CAD build for the part. Positions are in the model's coordinates, mm. A direction names the side the tool comes from. Coordinates: 2 decimals unless noted, no trailing zeros. Write each loop counter-clockwise with the first axis right and the second up, starting at its lowest first coordinate (ties: lowest second). Pieces come first, ordered by that corner, then holes. Notation, with made-up numbers: (-38.75, 65) - (6.25, 65) arc R24 ccw to (6.25, 76) - close; hole circle Ø4 at (-37.5, 79). An arc over 180 degrees is marked (long way). One line per question, with ' | ' between items. Start each with the question number.
1. Which spindle directions (+Z, -Z, +X, -X, +Y, -Y) get a long thin tool onto all of the face, cutting with end or side? Do faces 1 (the flat face through (-90, 25, -5)), 2 (the flat face through (8, 10, -55)), 3 (the flat face through (40, 5, -26)), 4 (the flat face through (-40, 5, -26)), 5 (the flat face through (90, 25, -5)). Say none if no direction does.
2. Flat gauge pins, fed straight in: P1, Ø12, axis at x = -20.5, z = -42, coming from the +Y side; P2, Ø6, axis at x = -5, z = -49.5, coming from the +Y side; P3, Ø3, axis at y = 4.5, z = -26.5, coming from the +X side; P4, Ø4, axis at x = -24.5, y = 17, coming from the -Z side. Where does each tip first touch, or does it go through?
3. Probe line 1 (X direction, y = 7, z = -42); line 2 (Z direction, x = 51.5, y = 28.5); line 3 (Y direction, x = 2, z = -70). List the from-to ranges inside material, lowest first.
4. Band-saw the part on A-A, the plane x = 0. Write the cut outline in (y, z), then the cut area to 3 significant figures.
5. Band-saw the part on B-B, the plane y = 7. Write the cut outline in (x, z).
6. Band-saw the part on D-D, the plane x = 24. Write the cut outline in (y, z).
7. Band-saw the part on C-C, the plane z = -34. Write the cut outline in (x, y).
8. Two-plate mould, pull along Z, no slides. Class faces 6 (the flat face through (-1, 25, 0)), 7 (the flat face through (-1, 50, -5)), 8 (the cylindrical face through (0.88, 4.93, -82.49)), 9 (the cylindrical face through (8.45, 4.93, -51.71)): +Z half, -Z half, draft (parallel to the pull), parting line (faces both ways), or undercut.
from build123d import *

# Parameters (mm, degrees)
SKETCH1_R           = 12.5
BOSS_EXTRUDE1_DEPTH = 10
SKETCH2_W           = 180
SKETCH2_H           = 50
BOSS_EXTRUDE2_DEPTH = 10


with BuildPart() as part:
    # Sketch1 → Boss-Extrude1 (new body)
    with BuildSketch(Plane(origin=(0, 0, 0), x_dir=(1, 0, 0), z_dir=(0, 1, 0))):
        with BuildLine():
            Line((-40, 0), (40, 0))
            Line((40, 0), (40, 42.5))
            ThreePointArc((40, 42.5), (0, 82.5), (-40, 42.5))
            Line((-40, 42.5), (-40, 0))
        make_face()
        with Locations(Location((0, 42.5, 0), (0, 0, 270))):
            Circle(SKETCH1_R, mode=Mode.SUBTRACT)
    extrude(amount=BOSS_EXTRUDE1_DEPTH)

    # Sketch2 → Boss-Extrude2 (add)
    with BuildSketch(Plane.XY):
        with Locations((0, 25)):
            Rectangle(SKETCH2_W, SKETCH2_H)
    extrude(amount=-BOSS_EXTRUDE2_DEPTH)


solid = part.part
Filled in:
1) face 1: +Z, -Z, -X, +Y, -Y | face 2: -Z, +X, -X, +Y | face 3: -Z, +X, +Y, -Y | face 4: -Z, -X, +Y, -Y | face 5: +Z, -Z, +X, +Y, -Y
2) P1: stops at y = 10 | P2: passes through | P3: stops at x = 40 | P4: stops at z = -10
3) line 1: x = -40 to -12.49, 12.49 to 40 | line 2: z = -10 to 0 | line 3: y = 0 to 10
4) outline: (0, -82.5) - (10, -82.5) - (10, -55) - (0, -55) - close; (0, -30) - (10, -30) - (10, -10) - (50, -10) - (50, 0) - (0, 0) - close | area: 975 mm²
5) outline: (-90, -10) - (-40, -10) - (-40, -42.5) arc R40 ccw to (40, -42.5) - (40, -10) - (90, -10) - (90, 0) - (-90, 0) - close; hole circle Ø25 at (0, -42.5)
6) outline: (0, -74.5) - (10, -74.5) - (10, -10) - (50, -10) - (50, 0) - (0, 0) - close
7) outline: (-40, 0) - (-9.17, 0) - (-9.17, 10) - (-40, 10) - close; (9.17, 0) - (40, 0) - (40, 10) - (9.17, 10) - close
8) face 6: +Z half | face 7: draft | face 8: -Z half | face 9: undercut
